Verification items for this drawing (mm, ordinates from the low corner). Round coordinates to 2 decimals unless told otherwise and drop trailing zeros. Order: outer loops, then holes, each group sorted by start corner. A loop starts at its lowest first (then second) coordinate and runs counter-clockwise, first axis right, second up. Notation, with made-up numbers: (79, 57) -> (127, 57) arc R16 ccw to (127, 81) -> close; hole circle Ø7 at (-23, 70.25). An arc over 180 degrees is marked (long way). Answer in a Markdown table with one row per item.
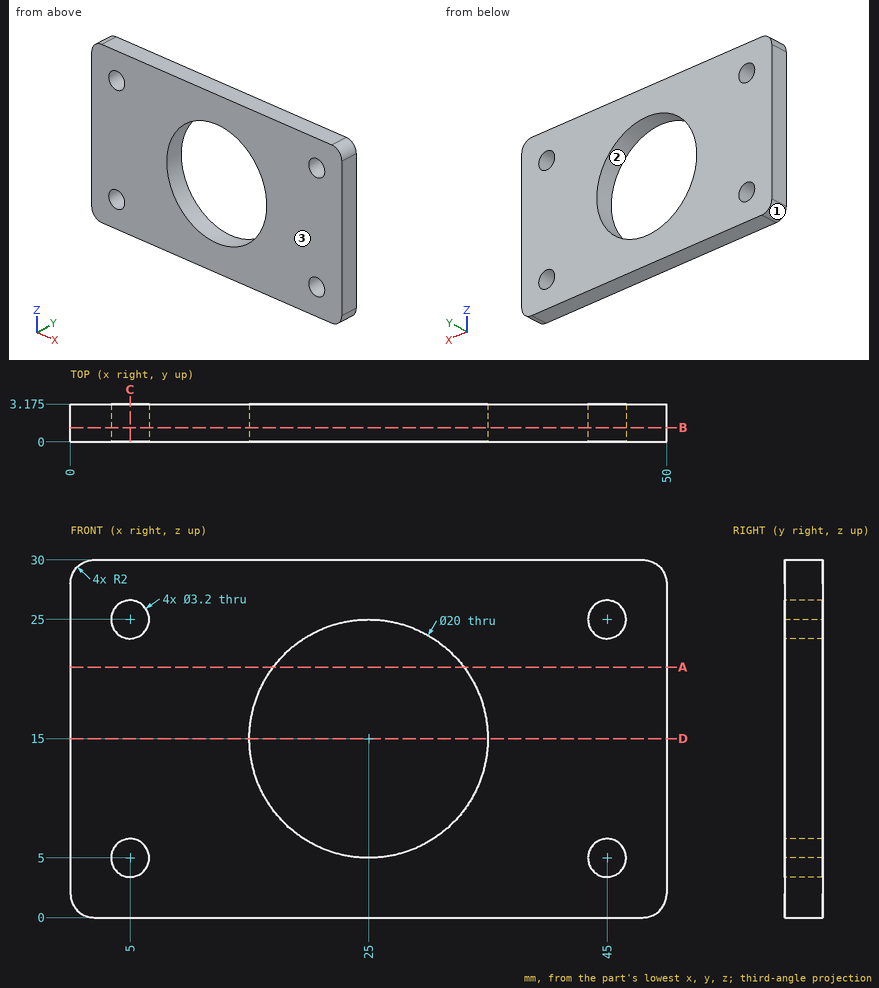
Item 1: Cross-section at C-C (x = 5). Record the boundary of the cut face in (y, z) (3 decimals), and give its area (3 significant figures).
Result sheet:
| item | result |
|---|---|
| outline | (0, 0) -> (3.175, 0) -> (3.175, 3.4) -> (0, 3.4) -> close; (0, 6.6) -> (3.175, 6.6) -> (3.175, 23.4) -> (0, 23.4) -> close; (0, 26.6) -> (3.175, 26.6) -> (3.175, 30) -> (0, 30) -> close |
| area | 74.9 mm^2 |
Item 2: Cross-section at A-A (z = 21). Record the boundary of the cut face in (x, y) (3 decimals), and give its area (3 significant figures).
Result sheet:
| item | result |
|---|---|
| outline | (0, 0) -> (17, 0) -> (17, 3.175) -> (0, 3.175) -> close; (33, 0) -> (50, 0) -> (50, 3.175) -> (33, 3.175) -> close |
| area | 108 mm^2 |
Item 3: Scan lines: line 1 (Z direction, x = 5, y = 0.8); line 2 (Z direction, x = 4, y = 3); line 3 (Z direction, x = 19, y = 1.4). Record each from-to range of solid material in increasing order. Write a range as [from, to].
Result sheet:
| item | result |
|---|---|
| line 1 | z = [0, 3.4], [6.6, 23.4], [26.6, 30] |
| line 2 | z = [0, 3.75], [6.25, 23.75], [26.25, 30] |
| line 3 | z = [0, 7], [23, 30] |
Item 4: Mould release check, pull along X, two halves, no side actions. Record for the marked faces 1, 2 and 3: pulls with the +X half, pulls with the -X half, needs draft (parallel to the pull), parting line crosses it, or undercut.
Result sheet:
| item | result |
|---|---|
| face 1 | pulls with the -X half |
| face 2 | undercut |
| face 3 | needs draft |
Item 5: Cross-section at D-D (z = 15). Record the boundary of the cut face in (x, y) (3 decimals), and give its area (4 significant figures).
Result sheet:
| item | result |
|---|---|
| outline | (0, 0) -> (15, 0) -> (15, 3.175) -> (0, 3.175) -> close; (35, 0) -> (50, 0) -> (50, 3.175) -> (35, 3.175) -> close |
| area | 95.25 mm^2 |
Item 6: Cross-section at B-B (y = 1.2). Record the boundary of the cut face in (x, z), and give its area (3 significant figures).
Result sheet:
| item | result |
|---|---|
| outline | (0, 2) arc R2 ccw to (2, 0) -> (48, 0) arc R2 ccw to (50, 2) -> (50, 28) arc R2 ccw to (48, 30) -> (2, 30) arc R2 ccw to (0, 28) -> close; hole circle Ø3.2 at (5, 5); hole circle Ø3.2 at (5, 25); hole circle Ø20 at (25, 15); hole circle Ø3.2 at (45, 5); hole circle Ø3.2 at (45, 25) |
| area | 1,150 mm^2 |
Item 7: Depth check by flat-ended pin: P1, Ø10, axis at x = 25, z = 9.5, coming from the -Y side. Enter the tip coordinate at first touch or a pass-through.
Result sheet:
| item | result |
|---|---|
| P1 | stops at y = 0 |
